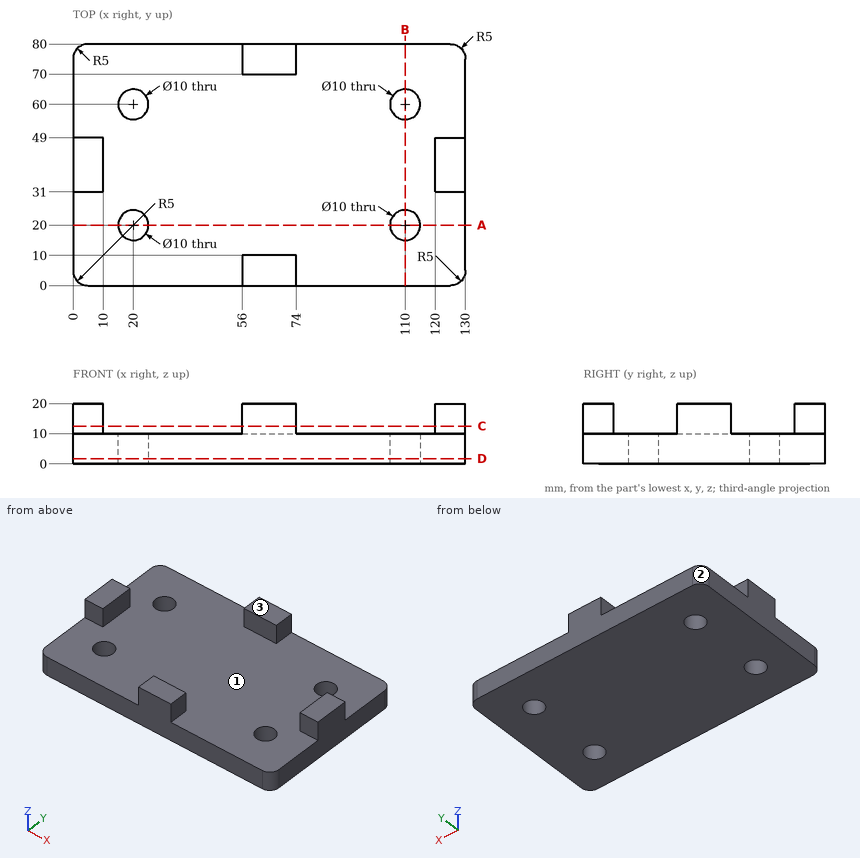
Design review of the part shown in the three views and the two pictorial views. Dimensions are in mm from the part's minimum x, y and z. Give positions to 0.01 mm unless a question says otherwise; leave off trailing zeros. Order: outer loops, then holes, each group sorted by start corner. A loop starts at its lowest first (then second) coordinate and runs counter-clockwise, first axis right, second up. Notation, with made-up numbers: (63, 55) -> (106, 55) arc R20 cw to (106, 79) -> close; hole circle Ø4 at (68.25, 79.5). An arc over 180 degrees is marked (long way). Write each question's results on one line, items separated by ' | '. Start each with the question number.
Q1. For pin 1 (2 mm diameter, centred on x = 31.5, y = 46.5, fed in from +Z); pin 2 (3 mm diameter, centred on y = 7.5, z = 17, fed in from +X); pin 3 (3 mm diameter, centred on y = 73.5, z = 16.5, fed in from -X), all flat-tipped, find the tip position at first contact; note any pin that passes through.
Q2. Wall thickness on L1, parallel to Y at x = 20, z = 3.75; L2, parallel to X at y = 21, z = 6.25; L3, parallel to Z at x = 25.5, y = 68: over which ranges is each line inside the solid? List them lowest first. Write a range as from..to.
Q3. Add section C-C on z = 12.5. Give the boundary of the cut face in (x, y).
Q4. Add section A-A on y = 20. Give the boundary of the cut face in (x, z).
Q5. Add section D-D on z = 1.75. Give the boundary of the cut face in (x, y).
Q6. Add section B-B on x = 110. Give the boundary of the cut face in (y, z), and give its area (3 significant figures).
Q7. Mouldability with a two-part tool opening along X and no side actions: class the marked faces 1, 2 and 3 as +X half, -X half, draft (parallel to the pull), parting line (faces both ways), or undercut.
Found:
1) pin 1: stops at z = 10 | pin 2: stops at x = 74 | pin 3: stops at x = 56
2) L1: y = 0..15, 25..55, 65..80 | L2: x = 0..15.1, 24.9..105.1, 114.9..130 | L3: z = 0..10
3) outline: (0, 31) -> (10, 31) -> (10, 49) -> (0, 49) -> close; (56, 0) -> (74, 0) -> (74, 10) -> (56, 10) -> close; (56, 70) -> (74, 70) -> (74, 80) -> (56, 80) -> close; (120, 31) -> (130, 31) -> (130, 49) -> (120, 49) -> close
4) outline: (0, 0) -> (15, 0) -> (15, 10) -> (0, 10) -> close; (25, 0) -> (105, 0) -> (105, 10) -> (25, 10) -> close; (115, 0) -> (130, 0) -> (130, 10) -> (115, 10) -> close
5) outline: (0, 5) arc R5 ccw to (5, 0) -> (125, 0) arc R5 ccw to (130, 5) -> (130, 75) arc R5 ccw to (125, 80) -> (5, 80) arc R5 ccw to (0, 75) -> close; hole circle Ø10 at (20, 20); hole circle Ø10 at (20, 60); hole circle Ø10 at (110, 20); hole circle Ø10 at (110, 60)
6) outline: (0, 0) -> (15, 0) -> (15, 10) -> (0, 10) -> close; (25, 0) -> (55, 0) -> (55, 10) -> (25, 10) -> close; (65, 0) -> (80, 0) -> (80, 10) -> (65, 10) -> close | area: 600 mm2
7) face 1: undercut | face 2: -X half | face 3: draft
